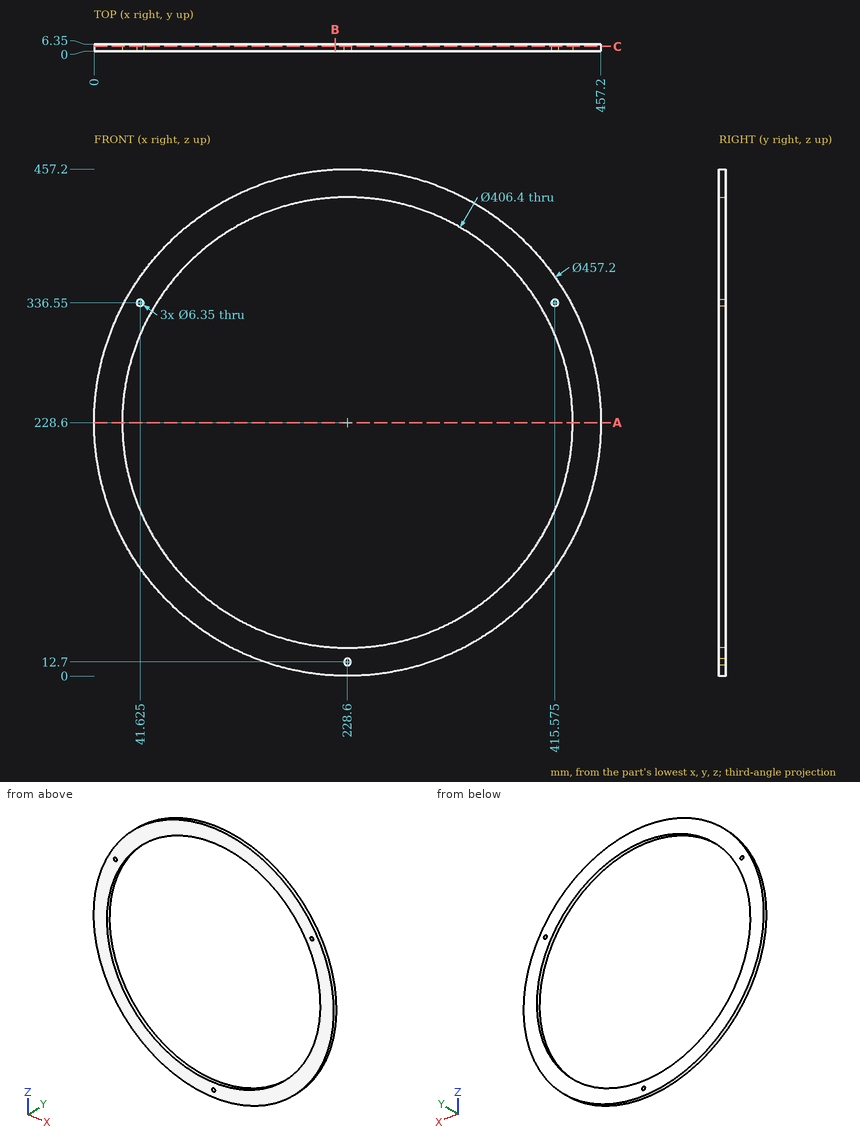
Check sheet for the drawn part. Datum: minimum x, y, z corner. Units: mm. Give positions to 0.01 mm unless a question says otherwise; leave off trailing zeros. Order: outer loops, then holes, each group sorted by start corner. A loop starts at its lowest first (then second) coordinate and runs counter-clockwise, first axis right, second up.
1. Depth check by flat-ended pin: pin 1 (5 mm diameter, centred on x = 41.63, z = 336.55, fed in from -Y); pin 2 (2 mm diameter, centred on y = 5, z = 352, fed in from +X); pin 3 (2 mm diameter, centred on x = 312, y = 5.5, fed in from -Z). Enter the tip coordinate at first touch or a pass-through.
Completed:
pin 1: passes through
pin 2: stops at x = 421.67
pin 3: stops at z = 15.37
2. Sectioned sample at C-C (y = 4.25). Record the boundary of the cut face in (x, z) (3 decimals), then the cut area to 3 significant figures.
Completed:
outline: circle Ø457.2 at (228.6, 228.6); hole circle Ø406.4 at (228.6, 228.6); hole circle Ø6.35 at (41.625, 336.55); hole circle Ø6.35 at (228.6, 12.7); hole circle Ø6.35 at (415.575, 336.55)
area: 34,400 mm2
3. Sectioned sample at A-A (z = 228.6). Record the boundary of the cut face in (x, y), then the cut area to 3 significant figures.
Completed:
outline: (0, 0) - (25.4, 0) - (25.4, 6.35) - (0, 6.35) - close; (431.8, 0) - (457.2, 0) - (457.2, 6.35) - (431.8, 6.35) - close
area: 323 mm2
4. Scan lines: line 1 (X direction, y = 2.25, z = 228.6); line 2 (X direction, y = 4.25, z = 336.55); line 3 (Z direction, x = 315.5, y = 1). Record each from-to range of solid material in increasing order.
Completed:
line 1: x = 0 to 25.4, 431.8 to 457.2
line 2: x = 27.09 to 38.45, 44.8 to 56.45, 400.75 to 412.4, 418.75 to 430.11
line 3: z = 17.16 to 44.92, 412.28 to 440.04
5. Sectioned sample at B-B (x = 217.5). Record the boundary of the cut face in (y, z).
Completed:
outline: (0, 0.27) - (6.35, 0.27) - (6.35, 25.7) - (0, 25.7) - close; (0, 431.5) - (6.35, 431.5) - (6.35, 456.93) - (0, 456.93) - close
